Check sheet for the drawn part. Datum: minimum x, y, z corner. Units: mm. Coordinates: 2 decimals unless noted, no trailing zeros. Write each loop counter-clockwise with the first axis right and the second up, starting at its lowest first coordinate (ties: lowest second). Pieces come first, ordered by that corner, then holes. Notation, with made-up numbers: M -22,78.25 L 28,78.25 A27 cw 28,104.25 Z; hole C 37,-19 d1. An arc over 180 degrees is marked long. Answer in a Markdown table with one row per item.
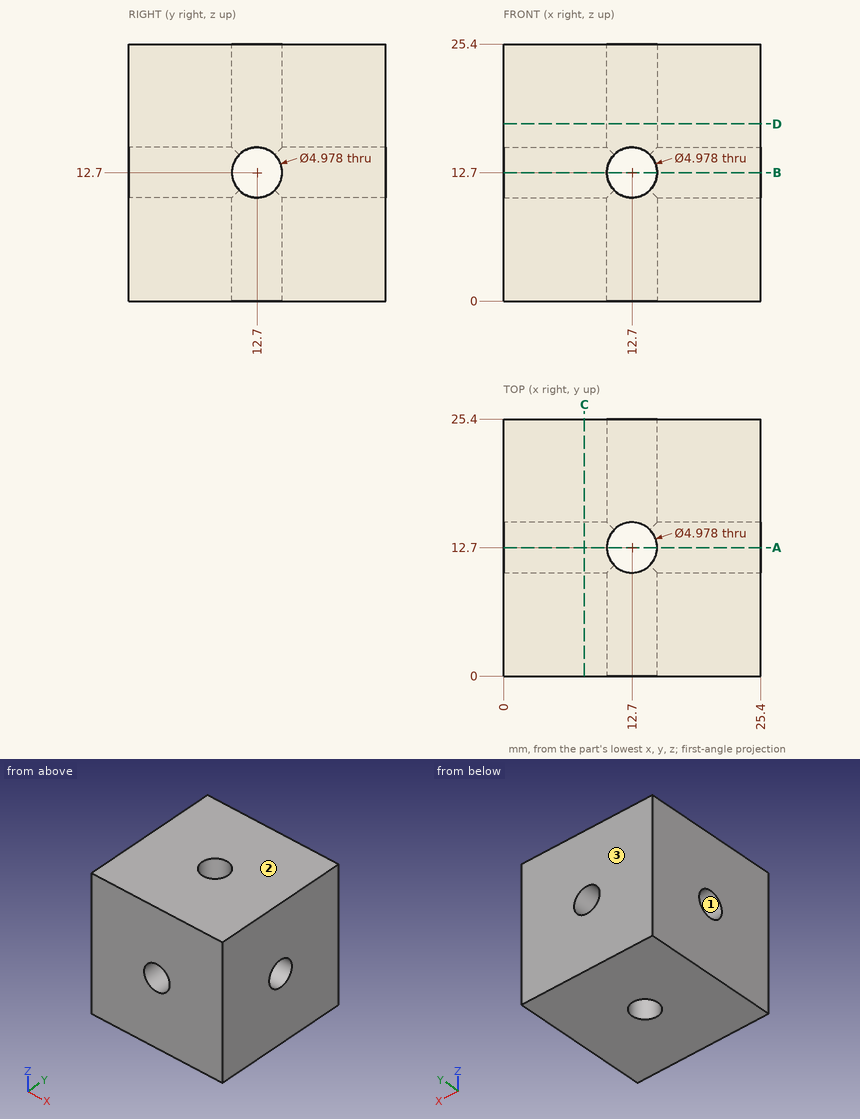
1) Sectioned sample at C-C (x = 8). Record the cut outline in (y, z), then the cut area to 3 significant figures.
Response values:
| item | result |
|---|---|
| outline | M 0,0 L 25.4,0 L 25.4,25.4 L 0,25.4 Z; hole C 12.7,12.7 d4.98 |
| area | 626 mm² |
2) Thickness scan on L1, parallel to Z at x = 12.7, y = 19. Record the ranges inside material, lowest first. Write a range as [from, to].
Response values:
| item | result |
|---|---|
| L1 | z = [0, 10.21], [15.19, 25.4] |
3) Release check for a two-part mould opening along Y. For the marked faces 1, 2 and 3 record: +Y half, -Y half, draft (parallel to the pull), parting line (faces both ways), or undercut.
Response values:
| item | result |
|---|---|
| face 1 | undercut |
| face 2 | draft |
| face 3 | +Y half |
4) Sectioned sample at A-A (y = 12.7). Record the cut outline in (x, z).
Response values:
| item | result |
|---|---|
| outline | M 0,0 L 10.21,0 L 10.21,10.21 L 0,10.21 Z; M 0,15.19 L 10.21,15.19 L 10.21,25.4 L 0,25.4 Z; M 15.19,0 L 25.4,0 L 25.4,10.21 L 15.19,10.21 Z; M 15.19,15.19 L 25.4,15.19 L 25.4,25.4 L 15.19,25.4 Z |
5) Depth check by flat-ended pin: pin 1 (5 mm diameter, centred on x = 4.5, z = 18.5, fed in from -Y); pin 2 (4.5 mm diameter, centred on x = 12.7, z = 12.7, fed in from +Y). Enter the tip coordinate at first touch or a pass-through.
Response values:
| item | result |
|---|---|
| pin 1 | stops at y = 0 |
| pin 2 | passes through |
